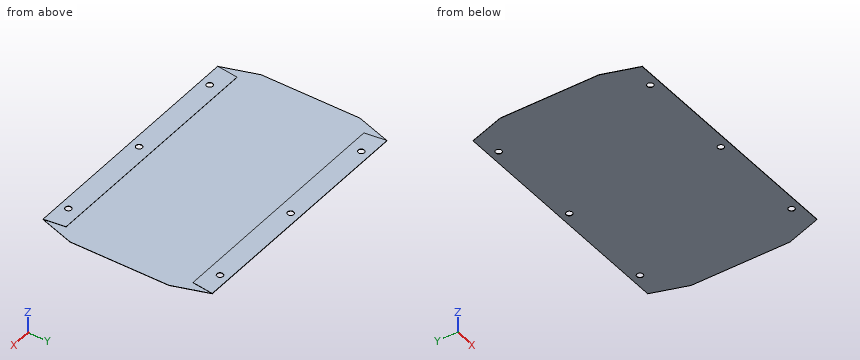
```python
from build123d import *

# Parameters (mm, degrees)
F1_DEPTH = 0.5
F3_DEPTH = 0.5
F4_R     = 8.788165
F5_DEPTH = 1.001


with BuildPart() as f1:
    # F0 (on Top) → F1 (new body)
    with BuildSketch(Plane.XY):
        Polygon((0, 0), (-700, 0), (-732.5, -100), (-732.5, -240), (-732.5, -380), (-700, -480), (0, -480), (32.5, -380), (32.5, -240), (32.5, -100), align=None)
    extrude(amount=F1_DEPTH)

    # F2 (on face) → F3 (join)
    with BuildSketch(Plane.XY.offset(0.5)):
        Polygon((0, 0), (-700, 0), (-692.5, -60), (-7.5, -60), align=None)
        Polygon((-692.5, -420), (-700, -480), (0, -480), (-7.5, -420), align=None)
    extrude(amount=F3_DEPTH)

    # F4 (on face) → F5 (cut, through all)
    with BuildSketch(Plane.XY.offset(1)):
        with Locations((-632.5, -25)):
            Circle(F4_R)
        with Locations((-632.5, -455)):
            Circle(F4_R)
        with Locations((-349.5, -25)):
            Circle(F4_R)
        with Locations((-349.5, -455)):
            Circle(F4_R)
        with Locations((-66.5, -25)):
            Circle(F4_R)
        with Locations((-66.5, -455)):
            Circle(F4_R)
    extrude(amount=-F5_DEPTH, mode=Mode.SUBTRACT)


solid = f1.part
```
Part model, mm, in its own coordinate system. Round coordinates to 2 decimals unless told otherwise and drop trailing zeros. Order: outer loops, then holes, each group sorted by start corner. A loop starts at its lowest first (then second) coordinate and runs counter-clockwise, first axis right, second up. Notation, with made-up numbers: M 72.5,50 L 91.5,50 A20 ccw 91.5,88 Z; hole C 66.5,-18.5 d3. An arc over 180 degrees is marked long. Answer in a Markdown table with one row per item. Add a question column.
Q1. Cut at C-C on x = -145. Give the cut face in (y, z).
Q2. Cut at D-D on y = -42. Give the cut face in (x, z).
Q3. Wall check: L1, parallel to Y at x = -66.5, z = 0.65; L2, parallel to Y at x = -605, z = 0.95; L3, parallel to Y at x = -342, z = 0.25. Give the ranges that are in metal, low to high. Write a range as from..to.
Q4. Cut at B-B on y = -455. Give the cut face in (x, z) (3 decimals), and give its area (3 significant figures).
Q5. Pin check, flat tips, straight feed: pin 1 (5 mm diameter, centred on x = -128, y = -67, fed in from +Z); pin 2 (14 mm diameter, centred on x = -349.5, y = -25, fed in from +Z). Stop position of each tip, or through.
Q6. Cut at A-A on x = -349.5. Give the cut face in (y, z), and give its area (3 significant figures).
Established:
| question | item | result |
|---|---|---|
| 1 | outline | M -480,0 L 0,0 L 0,1 L -60,1 L -60,0.5 L -420,0.5 L -420,1 L -480,1 Z |
| 2 | outline | M -713.65,0 L 13.65,0 L 13.65,0.5 L -5.25,0.5 L -5.25,1 L -694.75,1 L -694.75,0.5 L -713.65,0.5 Z |
| 3 | L1 | y = -480..-463.79, -446.21..-420, -60..-33.79, -16.21..0 |
| 3 | L2 | y = -480..-420, -60..0 |
| 3 | L3 | y = -480..-459.58, -450.42..-29.58, -20.42..0 |
| 4 | outline | M -708.125,0 L -641.288,0 L -641.288,1 L -696.875,1 L -696.875,0.5 L -708.125,0.5 Z; M -623.712,0 L -358.288,0 L -358.288,1 L -623.712,1 Z; M -340.712,0 L -75.288,0 L -75.288,1 L -340.712,1 Z; M -57.712,0 L 8.125,0 L 8.125,0.5 L -3.125,0.5 L -3.125,1 L -57.712,1 Z |
| 4 | area | 652 mm2 |
| 5 | pin 1 | stops at z = 0.5 |
| 5 | pin 2 | passes through |
| 6 | outline | M -480,0 L -463.79,0 L -463.79,1 L -480,1 Z; M -446.21,0 L -33.79,0 L -33.79,1 L -60,1 L -60,0.5 L -420,0.5 L -420,1 L -446.21,1 Z; M -16.21,0 L 0,0 L 0,1 L -16.21,1 Z |
| 6 | area | 265 mm2 |
